from build123d import *

# Parameters (mm, degrees)
F1_DEPTH = 70
F2_R     = 3
F3_DEPTH = 115


with BuildPart() as f1:
    # F0 (on Front) → F1 (new body)
    with BuildSketch(Plane.XZ):
        Polygon((-7.960861, 26.540911), (-7.960861, 16.540911), (-6.33612, 16.540911), (-4.585601, 14.040911), (0.414399, 14.040911), (2.164918, 16.540911), (5.414399, 16.540911), (5.414399, -23.459089), (2.164918, -23.459089), (0.414399, -20.959089), (-4.585601, -20.959089), (-6.33612, -23.459089), (-7.960861, -23.459089), (-7.960861, -33.459089), (17.039139, -33.459089), (17.039139, 26.540911), align=None)
    extrude(amount=F1_DEPTH)

    # F2 (on face) → F3 (join)
    with BuildSketch(Plane.YZ.offset(17.039139)):
        with Locations((-65, -15.459089)):
            Circle(F2_R)
        with Locations((-5, -15.459089)):
            Circle(F2_R)
    extrude(amount=F3_DEPTH)


solid = f1.part
The listing builds one solid part. Answer for the finished solid, in the listing's coordinates (mm). A direction names the side the tool comes from. Coordinates: 2 decimals unless noted, no trailing zeros. Loops run counter-clockwise (first coordinate to the right, second up) from the corner with the lowest first, then second, coordinate; pieces in that order, holes last.
1) Find the intervals of material crossed by L1, parallel to X at y = -17, z = -24.5; L2, parallel to X at y = -28.5, z = 7; L3, parallel to Z at x = 0, y = -52, in increasing order.
2) Find section A-A on y = -34. Write down the section's boundary in (x, z).
3) Determine the mould class of faces 4 (the face through (4, -35, 16.541)), 5 (the face through (73.73, -67.21, -13.43)), 6 (the face through (132.039, -5, -15)), 7 (the face through (4, -35, -23.459)) for opening direction Z: pulls with the +Z half, pulls with the -Z half, needs draft (parallel to the pull), parting line crosses it, or undercut.
4) A tool of negligible diameter and unlimited length cuts with its end or side. For faces 1 (the face through (73.734, -5.391, -12.485)), 2 (the face through (4, -35, -33.459)), 3 (the face through (-2, -35, -20.959)), from which of +Z, -Z, +X, -X, +Y, -Y can it reach the whole face along a straight path? Write none if from no direction.
5) Find section B-B on x = 122. Write down the section's boundary in (y, z).
6) Find section C-C on z = 23. Write down the section's boundary in (x, y).
7) Find section D-D on y = -65. Write down the section's boundary in (x, z).
8) Flat-ended cylindrical pins translate along their axes: pin 1 Ø4 at (y, z) = (-31, -8.5) entering from +X; pin 2 Ø20 at (y, z) = (-35.5, -9.5) entering from -X. Find the tip coordinate at first contact, or state that the pin passes through.
Values:
1. L1: x = -7.96 to 17.04
1. L2: x = 5.41 to 17.04
1. L3: z = -33.46 to -20.96, 14.04 to 26.54
2. outline: (-7.96, -33.46) - (17.04, -33.46) - (17.04, 26.54) - (-7.96, 26.54) - (-7.96, 16.54) - (-6.34, 16.54) - (-4.59, 14.04) - (0.41, 14.04) - (2.16, 16.54) - (5.41, 16.54) - (5.41, -23.46) - (2.16, -23.46) - (0.41, -20.96) - (-4.59, -20.96) - (-6.34, -23.46) - (-7.96, -23.46) - close
3. face 4: undercut
3. face 5: parting line crosses it
3. face 6: needs draft
3. face 7: undercut
4. face 1: +X
4. face 2: -Z, +X, -X, +Y, -Y
4. face 3: -X, +Y, -Y
5. outline: circle Ø6 at (-65, -15.46); circle Ø6 at (-5, -15.46)
6. outline: (-7.96, -70) - (17.04, -70) - (17.04, 0) - (-7.96, 0) - close
7. outline: (-7.96, -33.46) - (17.04, -33.46) - (17.04, -18.46) - (132.04, -18.46) - (132.04, -12.46) - (17.04, -12.46) - (17.04, 26.54) - (-7.96, 26.54) - (-7.96, 16.54) - (-6.34, 16.54) - (-4.59, 14.04) - (0.41, 14.04) - (2.16, 16.54) - (5.41, 16.54) - (5.41, -23.46) - (2.16, -23.46) - (0.41, -20.96) - (-4.59, -20.96) - (-6.34, -23.46) - (-7.96, -23.46) - close
8. pin 1: stops at x = 17.04
8. pin 2: stops at x = 5.41
